Can you work these out from the model? Positions are in its coordinate system, mm. Face numbers are marked on the shaded views. A direction names the side the tool comes from. Give positions to 0.01 mm unless a question says otherwise; leave off trailing zeros. Order: outer loops, then holes, each group sorted by start corner. A loop starts at its lowest first (then second) coordinate and runs counter-clockwise, first axis right, second up. Notation, with made-up numbers: (49.25, -5.75) -> (95.25, -5.75) arc R18 ccw to (95.25, 0.25) -> close; hole circle Ø1 at (45.25, 74). An arc over 180 degrees is marked (long way). Answer as CSV lines item,"result".
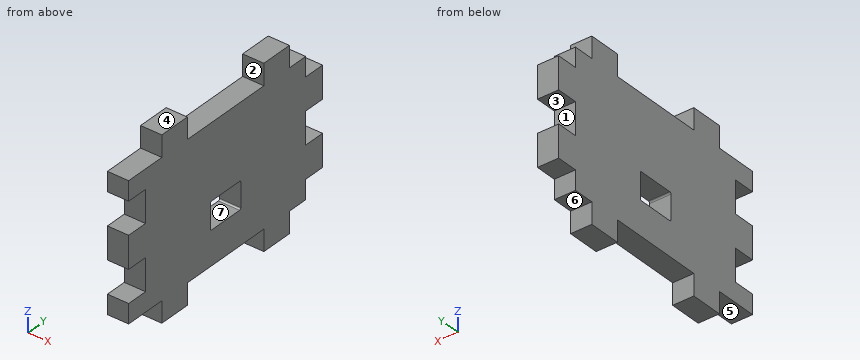
```python
from build123d import *

# Parameters (mm, degrees)
F0_W     = 76
F0_H     = 42
F1_DEPTH = 6.6
F2_W     = 10
F2_H     = 6.6
F3_DEPTH = 6.6
F4_W     = 6.6
F4_H     = 6
F4_H_2   = 10
F5_DEPTH = 6.6
F6_W     = 12
F6_H     = 8.5
F7_DEPTH = 6.6
F8_R     = 0.5


with BuildPart() as f1:
    # F0 (on Right) → F1 (new body)
    with BuildSketch(Plane.YZ):
        Rectangle(F0_W, F0_H)
    extrude(amount=F1_DEPTH)

    # F2 (on face) → F3 (join)
    with BuildSketch(Plane.YZ.offset(6.6)):
        with Locations((-20, 24.3)):
            Rectangle(F2_W, F2_H)
        with Locations((20, 24.3)):
            Rectangle(F2_W, F2_H)
        with Locations((20, -24.3)):
            Rectangle(F2_W, F2_H)
        with Locations((-20, -24.3)):
            Rectangle(F2_W, F2_H)
    extrude(amount=-F3_DEPTH)

    # F4 (on face) → F5 (cut, through all)
    with BuildSketch(Plane.YZ.offset(6.6)):
        with Locations((34.7, 18)):
            Rectangle(F4_W, F4_H)
        with Locations((34.7, -18)):
            Rectangle(F4_W, F4_H)
        with Locations((34.7, 0)):
            Rectangle(F4_W, F4_H_2)
        with Locations((-34.7, 10)):
            Rectangle(F4_W, F4_H_2)
        with Locations((-34.7, -10)):
            Rectangle(F4_W, F4_H_2)
    extrude(amount=-F5_DEPTH, mode=Mode.SUBTRACT)

    # F6 (on face) → F7 (cut, through all)
    with BuildSketch(Plane.YZ.offset(6.6)):
        with Locations((0, -6.25)):
            Rectangle(F6_W, F6_H)
    extrude(amount=-F7_DEPTH, mode=Mode.SUBTRACT)

    # F8
    f8_edges = [f1.edges().sort_by_distance(p)[0] for p in [
        (3.3, -6, -2),
        (3.3, 6, -2),
        (3.3, 6, -10.5),
        (3.3, -6, -10.5),
    ]]
    fillet(f8_edges, radius=F8_R)


solid = f1.part
```
Item 1: For the marked faces 5, 6 and 7, which set-ups out of +Z, -Z, +X, -X, +Y, -Y let a thin tool reach every point of the face, with its end or its side?
Numbers:
face 5,"-Z, +X, -X, -Y"
face 6,"-Z, +X, -X, +Y"
face 7,"+X, -X"
Item 2: Imagine slicing it at A-A, the plane z = -8. Please give me the cut outline in (x, y), then the cut area to 3 significant figures.
Numbers:
outline,"(0, -31.4) -> (6.6, -31.4) -> (6.6, -6) -> (0, -6) -> close; (0, 6) -> (6.6, 6) -> (6.6, 38) -> (0, 38) -> close"
area,"379 mm²"
Item 3: We'd pull the mould along Z, two halves only. Please class the marked faces 1, 2, 3 and 4: released by +Z, released by -Z, zero draft, split by the parting line, or undercut.
Numbers:
face 1,"undercut"
face 2,"zero draft"
face 3,"undercut"
face 4,"released by +Z"
Item 4: Please list where these lines run through material, in increasing order: line 1 along Y through (x, z) = (2.75, -7); line 2 along Z through (x, y) = (5.75, -3.5); line 3 along Y through (x, z) = (2.25, -25).
Numbers:
line 1,"y = -31.4 to -6, 6 to 38"
line 2,"z = -21 to -10.5, -2 to 21"
line 3,"y = -25 to -15, 15 to 25"
Item 5: Imagine slicing it at B-B, the plane y = -28. Please give me the cut outline in (x, z), then the cut area to 3 significant figures.
Numbers:
outline,"(0, -21) -> (6.6, -21) -> (6.6, 21) -> (0, 21) -> close"
area,"277 mm²"
Item 6: For pin 1 (3 mm diameter, centred on x = 5.5, z = 17.5, fed in from +Y); pin 2 (2 mm diameter, centred on x = 2, y = -32.5, fed in from +Z); pin 3 (3.5 mm diameter, centred on x = 4, y = -30.5, fed in from -Z), each with a flat end and sliding along its axis, tell me the tip position at first contact or that it passes through.
Numbers:
pin 1,"stops at y = 31.4"
pin 2,"stops at z = 21"
pin 3,"stops at z = -21"
Item 7: Imagine slicing it at C-C, the plane z = -17.5. Please give me the cut outline in (x, y).
Numbers:
outline,"(0, -38) -> (6.6, -38) -> (6.6, 31.4) -> (0, 31.4) -> close"
